Verification items for this drawing (mm, ordinates from the low corner). A direction names the side the tool comes from. Give positions to 0.01 mm unless a question says otherwise; leave off trailing zeros. Loops run counter-clockwise (first coordinate to the right, second up) from the corner with the lowest first, then second, coordinate; pieces in that order, holes last. Notation, with made-up numbers: (-0.75, 82) -> (16.25, 82) arc R14 cw to (16.25, 91) -> close; hole circle Ø9 at (54.5, 81). An arc over 180 degrees is marked (long way). Answer as a JSON object with one key per item and string values.
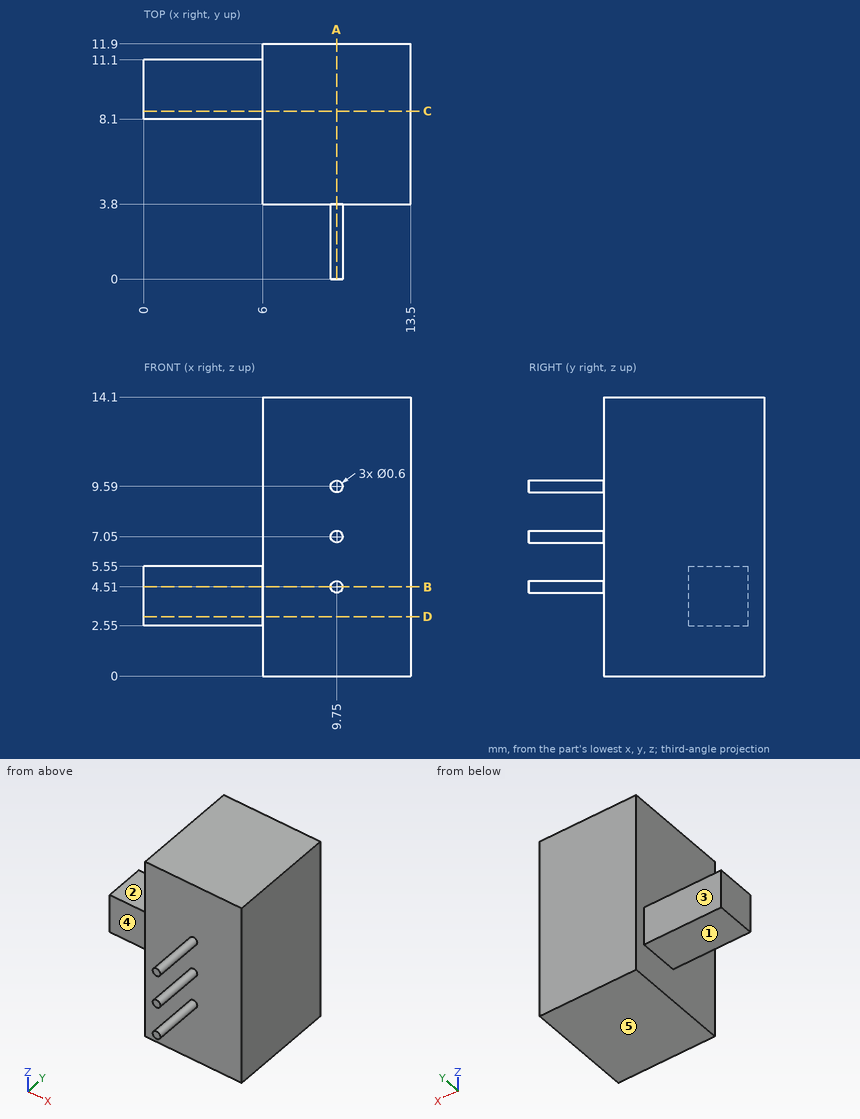
1) Section check D-D on z = 3. Record the cut outline in (x, y).
Geometry check:
{"outline": "(0, 8.1) -> (6, 8.1) -> (6, 3.8) -> (13.5, 3.8) -> (13.5, 11.9) -> (6, 11.9) -> (6, 11.1) -> (0, 11.1) -> close"}
2) Section check A-A on x = 9.75. Record the cut outline in (y, z), plus the area to 3 significant figures.
Geometry check:
{"outline": "(0, 4.21) -> (3.8, 4.21) -> (3.8, 0) -> (11.9, 0) -> (11.9, 14.1) -> (3.8, 14.1) -> (3.8, 9.89) -> (0, 9.89) -> (0, 9.29) -> (3.8, 9.29) -> (3.8, 7.35) -> (0, 7.35) -> (0, 6.75) -> (3.8, 6.75) -> (3.8, 4.81) -> (0, 4.81) -> close", "area": "121 mm2"}
3) Material ranges on line 1 along X through (y, z) = (11.5, 8); line 2 along Y through (x, z) = (8.25, 10.25); line 3 along Z through (x, y) = (1.5, 9), recorded low to high. Write a range as from..to.
Geometry check:
{"line 1": "x = 6..13.5", "line 2": "y = 3.8..11.9", "line 3": "z = 2.55..5.55"}
4) Section check B-B on z = 4.51. Record the cut outline in (x, y), plus the area to 3 significant figures.
Geometry check:
{"outline": "(0, 8.1) -> (6, 8.1) -> (6, 3.8) -> (9.45, 3.8) -> (9.45, 0) -> (10.05, 0) -> (10.05, 3.8) -> (13.5, 3.8) -> (13.5, 11.9) -> (6, 11.9) -> (6, 11.1) -> (0, 11.1) -> close", "area": "81.0 mm2"}
5) Tool access check on the marked faces 1, 2, 3, 4 and 5. Record the directions out of +Z, -Z, +X, -X, +Y, -Y that give a thin tool (end or side, any length) a straight path to the whole face; none if there is none.
Geometry check:
{"face 1": "-Z, -X, +Y, -Y", "face 2": "+Z, -X, +Y, -Y", "face 3": "+Z, -Z, -X, +Y", "face 4": "+Z, -Z, -X, -Y", "face 5": "-Z, +X, -X, +Y, -Y"}
6) Section check C-C on y = 8.5. Record the cut outline in (x, z).
Geometry check:
{"outline": "(0, 2.55) -> (6, 2.55) -> (6, 0) -> (13.5, 0) -> (13.5, 14.1) -> (6, 14.1) -> (6, 5.55) -> (0, 5.55) -> close"}
7) Depth check by flat-ended pin: P1, Ø1.5, axis at x = 1.5, y = 10, coming from the +Z side; P2, Ø3.5, axis at x = 2, z = 3.5, coming from the +Y side; P3, Ø2, axis at x = 6.5, z = 4, coming from the -Y side. Enter the tip coordinate at first touch or a pass-through.
Geometry check:
{"P1": "stops at z = 5.55", "P2": "stops at y = 11.1", "P3": "stops at y = 3.8"}
